Design review of the part built by this model. Coordinates are the model's own, in mm. A direction names the side the tool comes from. Coordinates: 2 decimals unless noted, no trailing zeros. Write each loop counter-clockwise with the first axis right and the second up, starting at its lowest first coordinate (ties: lowest second). Pieces come first, ordered by that corner, then holes.
Q1. Take a section at B-B (x = -6.5). Give the boundary of the cut face in (y, z).
Q2. Insertion check: pin 1 (1 mm diameter, centred on x = 9, y = -20, fed in from -Z); pin 2 (8.5 mm diameter, centred on x = -6, y = -20, fed in from -Z); pin 3 (6 mm diameter, centred on y = -14.5, z = 4.5, fed in from +X). Each pin has a flat end and moves straight along its axis. Give the tip position at first contact, or say it passes through.
Q3. Take a section at C-C (z = 1). Give the boundary of the cut face in (x, y), and give its area (3 significant figures).
Q4. Machinability: for faces 4 (the cylindrical face through (-0.35, -14.79, -4.694)), 5 (the cylindrical face through (15.132, -14.79, 0.027)), which of the approach directions +Z, -Z, +X, -X, +Y, -Y give a long, thin tool a straight path to every point of the face, cutting with its end or side? Answer none if there is none.
Q5. Mouldability with a two-part tool opening along X and no side actions: class faces 1 (the cylindrical face through (2.39, -14.79, 1.8)), 2 (the cylindrical face through (-16.01, -14.79, 0.37)), 3 (the flat face through (-2.4, -30, 2.1)) as pulls with the +X half, pulls with the -X half, needs draft (parallel to the pull), parting line crosses it, or undercut.
Q6. For probe 1 along Z at (x, y) = (3, -26.5); probe 2 along Z at (x, y) = (-12.5, -14.5); probe 3 along X at (y, z) = (-19.5, 1), list the stretches that pass through material, from the lowest coordinate up.
```python
from build123d import *

# Parameters (mm, degrees)
F2_DEPTH = 30
F3_DEPTH = 30.001


with BuildPart() as f2:
    # F1 (on Front) → F2 (new body)
    with BuildSketch(Plane.XZ):
        with BuildLine():
            ThreePointArc((-13.628092, 2.498427), (-13.282564, 2.458935), (-12.936335, 2.42617))
            ThreePointArc((-12.936335, 2.42617), (-13.279688, 2.486472), (-13.628092, 2.498427))
        make_face()
        with BuildLine():
            ThreePointArc((-1.995452, 5.049623), (-7.254227, 2.855159), (-12.936335, 2.42617))
            ThreePointArc((-12.936335, 2.42617), (-13.282564, 2.458935), (-13.628092, 2.498427))
            ThreePointArc((-13.628092, 2.498427), (-16.019104, 0.317987), (-14.255634, -2.395208))
            ThreePointArc((-14.255634, -2.395208), (-0.148783, -4.695078), (13.970789, -2.474639))
            ThreePointArc((13.970789, -2.474639), (16.110221, 0.163832), (13.644095, 2.499838))
            ThreePointArc((13.644095, 2.499838), (13.386962, 2.474302), (13.129503, 2.452288))
            ThreePointArc((13.129503, 2.452288), (7.36113, 2.887834), (1.995452, 5.049623))
            ThreePointArc((1.995452, 5.049623), (0, 5.691083), (-1.995452, 5.049623))
        make_face()
        with BuildLine():
            ThreePointArc((13.644095, 2.499838), (13.385567, 2.489395), (13.129503, 2.452288))
            ThreePointArc((13.129503, 2.452288), (13.386962, 2.474302), (13.644095, 2.499838))
        make_face()
    extrude(amount=F2_DEPTH)

    # F0 (on Front) → F3 (cut, through all)
    with BuildSketch(Plane.XZ):
        with BuildLine():
            Line((-2.934361, 1.4968), (-13.616795, 1.499978))
            ThreePointArc((-13.616795, 1.499978), (-15.108627, 0.221025), (-14.054368, -1.437234))
            ThreePointArc((-14.054368, -1.437234), (-14.014174, -1.448054), (-13.973971, -1.458842))
            ThreePointArc((-13.973971, -1.458842), (-7.047266, -2.835816), (0, -3.295535))
            Line((0, -3.295535), (0, 4.444465))
            ThreePointArc((0, 4.444465), (-1.516001, 3.827089), (-2.169382, 2.326253))
            ThreePointArc((-2.169382, 2.326253), (-2.403217, 1.774428), (-2.934361, 1.4968))
        make_face()
        with BuildLine():
            ThreePointArc((-13.973971, -1.458842), (-14.014174, -1.448054), (-14.054368, -1.437234))
            ThreePointArc((-14.054368, -1.437234), (-14.014319, -1.448596), (-13.973971, -1.458842))
        make_face()
        with BuildLine():
            Line((0, 4.444465), (0, -3.295535))
            ThreePointArc((0, -3.295535), (6.942098, -2.843865), (13.768233, -1.501997))
            ThreePointArc((13.768233, -1.501997), (15.131236, 0.059457), (13.633205, 1.491873))
            Line((13.633205, 1.491873), (2.844597, 1.495082))
            ThreePointArc((2.844597, 1.495082), (2.383494, 1.810344), (2.169382, 2.326253))
            ThreePointArc((2.169382, 2.326253), (1.516001, 3.827089), (0, 4.444465))
        make_face()
    extrude(amount=F3_DEPTH, mode=Mode.SUBTRACT)


solid = f2.part
```
Response:
1. outline: (-30, -4.23) - (0, -4.23) - (0, -2.9) - (-30, -2.9) - close; (-30, 1.5) - (0, 1.5) - (0, 3.05) - (-30, 3.05) - close
2. pin 1: stops at z = -3.88
2. pin 2: stops at z = -4.66
2. pin 3: stops at x = 15.62
3. outline: (-15.83, -30) - (-14.74, -30) - (-14.74, 0) - (-15.83, 0) - close; (14.74, -30) - (15.91, -30) - (15.91, 0) - (14.74, 0) - close
3. area: 67.5 mm2
4. face 4: -Z, +Y, -Y
4. face 5: +Y, -Y
5. face 1: undercut
5. face 2: pulls with the -X half
5. face 3: needs draft
6. probe 1: z = -4.59 to -3.21, 1.5 to 4.49
6. probe 2: z = -2.94 to -1.83, 1.5 to 2.39
6. probe 3: x = -15.83 to -14.74, 14.74 to 15.91
